Here's how the part is built. I have some questions about the finished solid (model axes, mm). Face numbers are marked on the shaded views. Round coordinates to 2 decimals unless told otherwise and drop trailing zeros. Loops run counter-clockwise (first coordinate to the right, second up) from the corner with the lowest first, then second, coordinate; pieces in that order, holes last. Notation, with made-up numbers: M 84,63.25 L 88,63.25 A20 cw 88,86.25 Z; hole C -31.75,82.25 d7. An arc over 180 degrees is marked long. Answer as a JSON object with one key per item and string values.
from build123d import *

# Parameters (mm, degrees)
SKETCH1_R           = 1.27
BOSS_EXTRUDE1_DEPTH = 6.35
FILLET1_R           = 7.62
FILLET2_R           = 2.54


with BuildPart() as part:
    # Sketch1 → Boss-Extrude1 (new body)
    with BuildSketch(Plane(origin=(0, 0, 0), x_dir=(1, 0, 0), z_dir=(0, 1, 0))):
        with BuildLine():
            Line((81.778930412, 21.890352424), (90.625383348, 37.130352424))
            ThreePointArc((90.625383348, 37.130352424), (36.535362906, 39.988317454), (0, 0))
            Line((0, 0), (-9.024498495, -42.227981756))
            Line((-9.024498495, -42.227981756), (3.372757994, -44.986498939))
            Line((3.372757994, -44.986498939), (12.397256489, -2.758517182))
            ThreePointArc((12.397256489, -2.758517182), (41.38133196, 25.629318142), (81.778930412, 21.890352424))
        make_face()
        with Locations(Location((-1.635035265, -36.315193683, 0), (0, 0, 270))):
            Circle(SKETCH1_R, mode=Mode.SUBTRACT)
    extrude(amount=BOSS_EXTRUDE1_DEPTH)

    # Fillet1
    fillet1_edges = [part.edges().sort_by_distance(p)[0] for p in [
        (90.625383348, 3.175, -37.130352424),
        (81.778930412, 3.175, -21.890352424),
    ]]
    fillet(fillet1_edges, radius=FILLET1_R)

    # Fillet2
    # the kernel refuses this fillet: 2.54 mm, written as the material it adds along each edge
    with BuildSketch(Plane(origin=(12.397256489, 0, 2.758517182), x_dir=(0.35622264546587595, 0, -0.9344011059803455), z_dir=(0, 1, 0))) as fillet2_piece_1:
        with BuildLine():
            CenterArc((0.195594606, -2.539994503), FILLET2_R, 89.880796264, 8.924440748)
            Line((-0.193218847, -0.029929942), (0, 0))
            ThreePointArc((0, 0), (0.100439533, 0.000104482), (0.200879066, 0))
        make_face()
    extrude(amount=6.35)
    # the kernel refuses this fillet: 2.54 mm, written as the material it takes off along each edge
    with BuildSketch(Plane(origin=(3.372757994, -6.403575534, 44.986498939), x_dir=(0.20898980989256036, 0, -0.9779178183063603), z_dir=(0, 1, 0))) as fillet2_2_piece_1:
        with BuildLine():
            CenterArc((FILLET2_R * 1.00843709196, FILLET2_R), FILLET2_R, 179.518623791, 90.481376209)
            Line((FILLET2_R * 0.00847238518745, FILLET2_R * 1.00840150095), (0, 0))
            Line((0, 0), (FILLET2_R * 1.00843709196, 0))
        make_face()
    extrude(amount=19.157151068, mode=Mode.SUBTRACT)
    with BuildSketch(Plane(origin=(-9.024498495, -6.296872706, 42.227981756), x_dir=(0.20898980989255983, 0, -0.9779178183063605), z_dir=(0, 1, 0))) as fillet2_2_piece_2:
        with BuildLine():
            CenterArc((FILLET2_R * 0.991633497, -FILLET2_R), FILLET2_R, 90, 89.518623791)
            Line((-FILLET2_R * 0.00833120976845, -FILLET2_R * 0.991598499049), (0, 0))
            Line((0, 0), (FILLET2_R * 0.991633497, 0))
        make_face()
    extrude(amount=18.943745412, mode=Mode.SUBTRACT)
    with BuildSketch(Plane(origin=(0, -0.288692893, 0), x_dir=(0.29511712664232287, 0, -0.9554610832275584), z_dir=(0, 1, 0))) as fillet2_2_piece_3:
        with BuildLine():
            CenterArc((0.11316262, -2.539998945), FILLET2_R, 89.947790074, 5.153611753)
            Line((-0.112690792, -0.010060164), (0, 0))
            ThreePointArc((0, 0), (0.057738579, 2.6307e-05), (0.115477157, 0))
        make_face()
    extrude(amount=6.927385787, mode=Mode.SUBTRACT)


solid = part.part
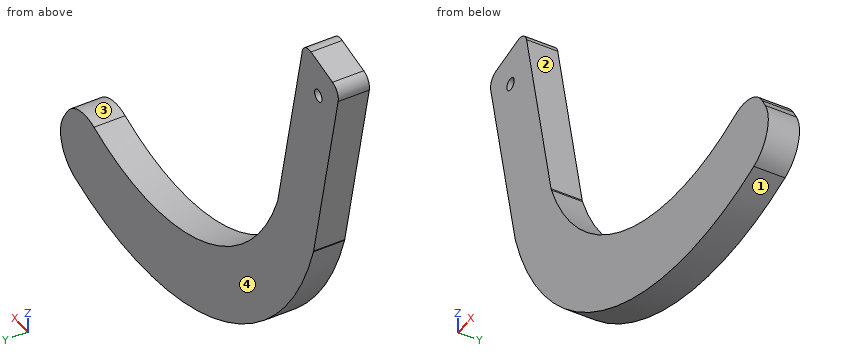
Item 1: I want a section at B-B on x = 51. List the corners of the cut face in (y, z) for me.
Solution:
{"outline": "M 0,-43.99 L 6.35,-43.99 L 6.35,-27.97 L 0,-27.97 Z"}
Item 2: If I drill on L1, parallel to X at y = 5, z = -13; L2, parallel to Z at x = 67.5, y = 2.5; L3, parallel to Z at x = 60, y = 4.5, over which ranges is the centre line in solid material (lowest first)? Write a range as from..to.
Solution:
{"L1": "x = 5.66..22.18", "L2": "z = -44.34..-27.38", "L3": "z = -44.72..-28.35"}
Item 3: We'd pull the mould along X, two halves only. Please class the marked faces 1, 2, 3 and 4: +X half, -X half, draft (parallel to the pull), parting line (faces both ways), or undercut.
Solution:
{"face 1": "parting line", "face 2": "+X half", "face 3": "undercut", "face 4": "draft"}
Item 4: I want a section at C-C on z = -23. List the corners of the cut face in (x, y) for me.
Solution:
{"outline": "M 12.8,0 L 35.33,0 L 35.33,6.35 L 12.8,6.35 Z"}
Item 5: I want a section at A-A on y = 5. List the corners of the cut face in (x, z) for me, plus the area to 3 significant figures.
Solution:
{"outline": "M -8.5,39.76 L -0.02,0.11 A2.54 ccw 0.03,-0.11 A63.36 ccw 82.44,-40.82 A7.62 ccw 86.4,-29.84 L 85.34,-28.03 A7.62 ccw 75.86,-24.8 A48.28 cw 12.47,2.57 A2.54 cw 12.36,2.95 L 3.91,42.48 A2.54 ccw 0.87,44.43 L -6.57,42.78 A2.54 ccw Z; hole C -1.64,36.32 d2.54", "area": "1,990 mm2"}
